Model file for the job. Use its own axes, mm. Coordinates: 2 decimals unless noted, no trailing zeros. Write each loop counter-clockwise with the first axis right and the second up, starting at its lowest first coordinate (ties: lowest second). Pieces come first, ordered by that corner, then holes.
Q1. Band-saw the part on C-C, the plane z = -235. Write the cut outline in (x, y), plus the area to 3 significant figures.
Q2. Drill centre lines: probe 1 along X at (y, z) = (4.6, -265.5); probe 2 along X at (y, z) = (3.85, -193.5). Where is each one in solid material? Low to high.
Q3. Pin check, flat tips, straight feed: P1, Ø1.8, axis at y = 2, z = -249, coming from the -X side; P2, Ø3, axis at y = 3.5, z = -189.5, coming from the -X side; P3, Ø4, axis at x = 0, z = -288.984, coming from the +Y side. Stop position of each tip, or through.
Q4. Band-saw the part on A-A, the plane y = 3.6. State how many separate pieces and enclosed holes the cut face has, plus the area to 3 significant figures.
Q5. Band-saw the part on B-B, the plane x = 0. Write the cut outline in (y, z) (3 decimals), plus the area to 3 significant figures.
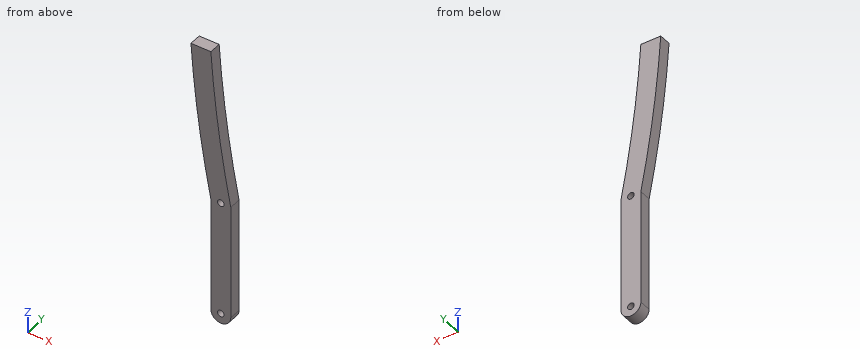
Autodesk Inventor part; units mm, degrees
ref_plane "YZ Plane" through (0, 0, 0) normal (1, 0, 0) x (0, 1, 0)
ref_plane "XZ Plane" through (0, 0, 0) normal (0, 1, 0) x (-1, 0, 0)
ref_plane "XY Plane" through (0, 0, 0) normal (0, 0, 1) x (1, 0, 0)
sketch "Sketch1" plane through (0, 0, 0) normal (0, 1, 0) x (-1, 0, 0)
  line L0 (0, 0) -> (0, -288.984) construction
  line L1 (5, 0) -> (5, -288.984)
  line L2 (-5, -288.984) -> (-5, 0)
  arc A0 (5, 0) -> (-5, 0) centre (0, 0) ccw
  arc A1 (-5, -288.984) -> (5, -288.984) centre (0, -288.984) ccw
  circle A2 centre (0, 0) radius 1.65
  circle A3 centre (0, -288.984) radius 1.65
  circle A4 centre (0, -231.585) radius 1.65
  arc A5 (-5, -231.585) -> (-5, 0) centre (-593.7207, -115.7925) ccw
  arc A6 (5, -231.585) -> (5, 0) centre (-583.7207, -115.7925) ccw
  circle A7 centre (11.23, -122.909) radius 1.65
  point P0 (0, -144.492)
  dimension "d0" = 3.3
  dimension "d1" = 3.3
  dimension "d2" = 10
  dimension "d3" = 288.984
  dimension "d14" = 3.3
  dimension "d15" = 231.585
  dimension "d18" = 600
  dimension "d19" = 600
  dimension "d20" = 3.3
  dimension "d21" = 122.909
extrude "Extrusion1" add sketch "Sketch1" along normal blind 6 contours L1 A1 L2 A5 | L1 A5 A6 | L1 A5 A0
sketch "Sketch2" plane through (0, 6, 0) normal (0, 1, 0) x (1, 0, 0)
  line L0 (-45.4801, 155.0502) -> (34.3076, 155.0502)
  line L1 (34.3076, 155.0502) -> (34.3076, -18.7731)
  line L2 (34.3076, -18.7731) -> (-45.4801, -18.7731)
  line L3 (-45.4801, -18.7731) -> (-45.4801, 155.0502)
  line L4 (-115.905, 316.254) -> (136.0777, 316.254)
  line L5 (136.0777, 316.254) -> (136.0777, -116.4724)
  line L6 (136.0777, -116.4724) -> (-115.905, -116.4724)
  line L7 (-115.905, -116.4724) -> (-115.905, 316.254)
  point P0 (0, 0)
extrude "Extrusion2" cut sketch "Sketch2" against normal blind 10 contours L0 L1 L2 L3
properties part number "Part_7_p2"
Answer sheet:
1. outline: (-5, 0) - (5, 0) - (5, 6) - (-5, 6) - close
1. area: 60.0 mm2
2. probe 1: x = -5 to 5
2. probe 2: x = -11.23 to -1.23
3. P1: stops at x = -5
3. P2: stops at x = -11.92
3. P3: stops at y = 6
4. separate pieces: 1
4. enclosed holes: 2
4. area: 1,360 mm2
5. outline: (0, -293.984) - (6, -293.984) - (6, -290.634) - (0, -290.634) - close; (0, -287.334) - (6, -287.334) - (6, -233.235) - (0, -233.235) - close; (0, -229.935) - (6, -229.935) - (6, -202.37) - (0, -202.37) - close
5. area: 510 mm2
